Could you check a few things on this drawing? It's one solid part, dimensions in mm from its lowest x, y, z. A direction names the side the tool comes from. Round coordinates to 2 decimals unless told otherwise and drop trailing zeros. Write each loop counter-clockwise with the first axis right and the second up, starting at its lowest first coordinate (ties: lowest second). Pieces come first, ordered by that corner, then holes. Notation, with made-up numbers: (-30, -11.75) -> (-12, -11.75) arc R33 ccw to (-12, 26.25) -> close; hole circle Ø10 at (57, -39.75). An arc over 180 degrees is marked (long way). Put each result on its own line as item: value. Start each with the question number.
1) Will these pins go through, and if not, where does the flat tip stop? P1, Ø12, axis at x = 9.5, z = 4, coming from the +Y side (1 decimal); P2, Ø8, axis at x = 22, y = 32, coming from the +Z side; P3, Ø6, axis at y = 6, z = 7, coming from the -X side.
2) I want a section at D-D, the plane x = 8. List the corners of the cut face in (y, z) for me (1 decimal).
3) I want a section at A-A, the plane x = 28. List the corners of the cut face in (y, z) for me, then the cut area to 3 significant figures.
4) We'd pull the mould along Y, two halves only. Please class the marked faces 1, 2 and 3: released by +Y, released by -Y, zero draft, split by the parting line, or undercut.
5) If I drill on line 1 along Y through (x, z) = (27.5, 24.25) (1 decimal); line 2 along Y through (x, z) = (28, 0.95); line 3 along Z through (x, y) = (45, 24.5), over which ranges is the centre line in solid material (lowest first)? Write a range as [from, to].
6) Which directions (+Z, -Z, +X, -X, +Y, -Y) give clear straight access to the entire face, cutting with the end or side of a thin tool? Please do the marked faces 4, 5, 6 and 7.
7) I want a section at B-B, the plane z = 20. List the corners of the cut face in (x, y) for me (1 decimal), then the cut area to 3 significant figures.
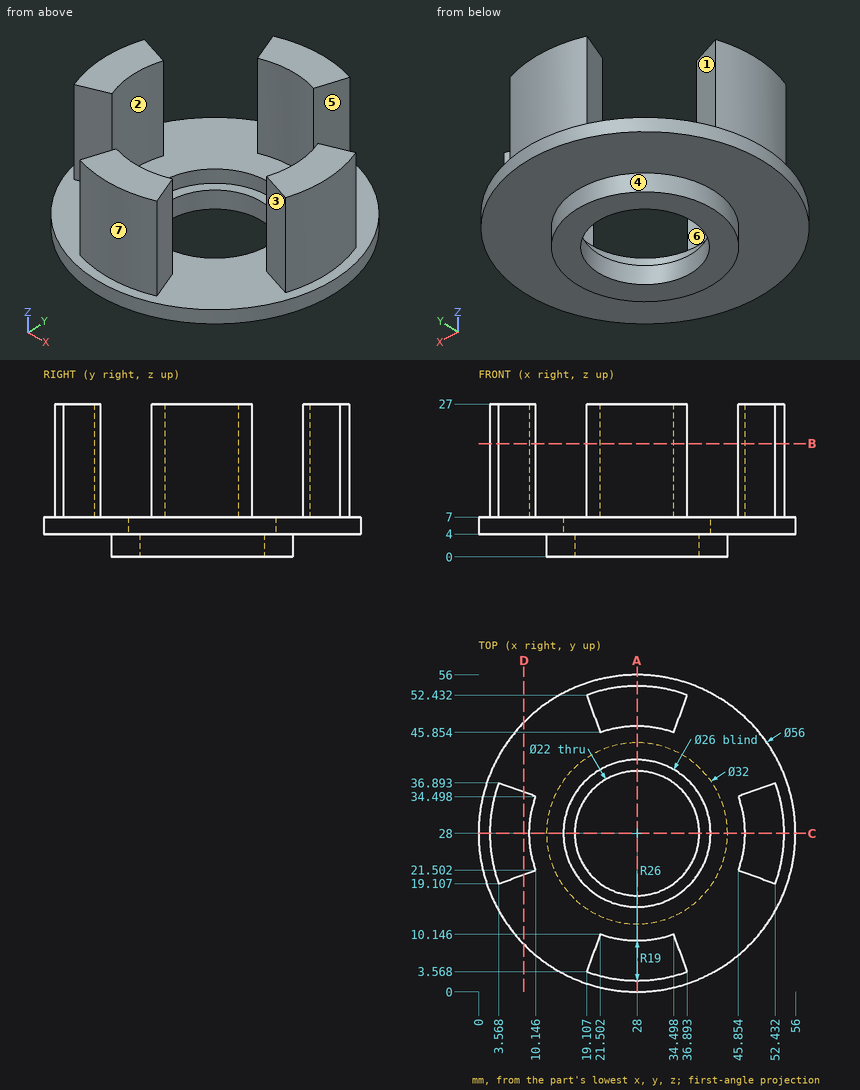
Findings:
1. P1: stops at y = 53.1
1. P2: stops at z = 4
1. P3: stops at x = 7.43
2. outline: (8.4, 4) -> (47.6, 4) -> (47.6, 7) -> (35.3, 7) -> (35.3, 27) -> (20.7, 27) -> (20.7, 7) -> (8.4, 7) -> close
3. outline: (0, 4) -> (12, 4) -> (12, 0) -> (17, 0) -> (17, 4) -> (15, 4) -> (15, 7) -> (9, 7) -> (9, 27) -> (2, 27) -> (2, 7) -> (0, 7) -> close; (39, 0) -> (44, 0) -> (44, 4) -> (56, 4) -> (56, 7) -> (54, 7) -> (54, 27) -> (47, 27) -> (47, 7) -> (41, 7) -> (41, 4) -> (39, 4) -> close
3. area: 410 mm2
4. face 1: released by +Y
4. face 2: undercut
4. face 3: released by -Y
5. line 1: y = [2, 9], [47, 54]
5. line 2: y = [12, 17], [39, 44]
5. line 3: z = [4, 7]
6. face 4: -Z
6. face 5: +Z, +X
6. face 6: +Z
6. face 7: +Z, -Y
7. outline: (3.6, 19.1) -> (10.1, 21.5) arc R19 cw to (10.1, 34.5) -> (3.6, 36.9) arc R26 ccw to start; (19.1, 3.6) arc R26 ccw to (36.9, 3.6) -> (34.5, 10.1) arc R19 cw to (21.5, 10.1) -> close; (19.1, 52.4) -> (21.5, 45.9) arc R19 cw to (34.5, 45.9) -> (36.9, 52.4) arc R26 ccw to start; (45.9, 21.5) -> (52.4, 19.1) arc R26 ccw to (52.4, 36.9) -> (45.9, 34.5) arc R19 cw to start
7. area: 440 mm2
